Autodesk Inventor part; units mm, degrees
ref_plane "YZ Plane" through (0, 0, 0) normal (1, 0, 0) x (0, 1, 0)
ref_plane "XZ Plane" through (0, 0, 0) normal (0, 1, 0) x (-1, 0, 0)
ref_plane "XY Plane" through (0, 0, 0) normal (0, 0, 1) x (1, 0, 0)
sketch "Sketch1" plane through (0, 0, 0) normal (0, 1, 0) x (-1, 0, 0)
  line L0 (-6, 0) -> (0, 0) construction
  line L1 (-27, 15) -> (-27, -15)
  line L2 (-27, 15) -> (-23, 15)
  line L3 (-27, -15) -> (-23, -15)
  line L4 (-5.8057, 1.5145) -> (-23, 6)
  line L5 (-5.8057, -1.5145) -> (-23, -6)
  arc A0 (-5.8057, -1.5145) -> (-5.8057, 1.5145) centre (-0.0058, 0) ccw
  line L6 (-23, 15) -> (-23, 6)
  line L7 (-23, -6) -> (-23, -15)
  dimension "d6" = 30
  dimension "d7" = 4
  dimension "d8" = 4
  dimension "d10" = 5.9944
extrude "Extrusion1" add sketch "Sketch1" along normal blind 762
properties part number "supportedLinearRail12mm_30inches"
The model under review builds one solid part; all positions refer to its coordinate system, in mm. A direction names the side the tool comes from. Round coordinates to 2 decimals unless told otherwise and drop trailing zeros. Loops run counter-clockwise (first coordinate to the right, second up) from the corner with the lowest first, then second, coordinate; pieces in that order, holes last. Notation, with made-up numbers: (-36.75, 12.5) -> (12.25, 12.5) arc R20 ccw to (12.25, 39.5) -> close; hole circle Ø9 at (20.25, 55.25). An arc over 180 degrees is marked (long way). Return JSON: item names as keys, results as strings.
(1) For faces 4 (the flat face through (14, 0, 0)), 5 (the flat face through (14.282, 375.666, -3.726)), list the 3-axis set-ups (+Z, -Z, +X, -X, +Y, -Y) from which the entire face can be reached by the end or side of a thin tool; tool diameter is ignored.
Solved:
{"face 4": "+Z, -Z, +X, -X, -Y", "face 5": "-Z, +Y, -Y"}
(2) The part is to be moulded in two halves that separate along X. For faces 1 (the flat face through (14.282, 375.666, 3.726)), 2 (the flat face through (14, 762, 0)), 3 (the flat face through (27, 376, 0)), say which applies: released by +X, released by -X, zero draft, split by the parting line, or undercut.
Solved:
{"face 1": "undercut", "face 2": "zero draft", "face 3": "released by +X"}
(3) Add section A-A on y = 394. Write out the cut boundary in (x, z).
Solved:
{"outline": "(5.81, -1.51) -> (23, -6) -> (23, -15) -> (27, -15) -> (27, 15) -> (23, 15) -> (23, 6) -> (5.81, 1.51) arc R5.99 ccw (long way) to start"}
(4) For pin 1 (2 mm diameter, centred on x = 8, y = 415.5, fed in from -Z); pin 2 (4.5 mm diameter, centred on y = 214.5, z = 10, fed in from -X); pin 3 (1 mm diameter, centred on x = 16.5, y = 180, fed in from +Z), all flat-tipped, find the tip position at first contact; note any pin that passes through.
Solved:
{"pin 1": "z = -2.35", "pin 2": "x = 23", "pin 3": "z = 4.43"}
(5) For line 1 (Z direction, x = -0.5, y = 130.5); line 2 (X direction, y = 159.5, z = -9); line 3 (Z direction, x = 6.5, y = 164), list the stretches that pass through material, from the lowest coordinate up.
Solved:
{"line 1": "-5.97 to 5.97", "line 2": "23 to 27", "line 3": "-1.7 to 1.7"}
(6) Add section B-B on x = -1. Write out the cut boundary in (y, z).
Solved:
{"outline": "(0, -5.91) -> (762, -5.91) -> (762, 5.91) -> (0, 5.91) -> close"}
